from build123d import *

# Parameters (mm, degrees)
F0_W     = 44.8449254036
F0_H     = 34.0256392956
F1_DEPTH = 330
F2_DEPTH = 900
F3_DEPTH = 600
F4_T     = -18
F6_W     = 48.9012300968
F6_H     = 42.5849854946
F7_DEPTH = 330
F8_DEPTH = 700
F9_DEPTH = 600
F10_T    = -18


with BuildPart() as f1:
    # F0 (on Front) → F1 (new body)
    with BuildSketch(Plane.XZ):
        with Locations((22.4224627018, 17.0128196478)):
            Rectangle(F0_W, F0_H)
    extrude(amount=F1_DEPTH)

    # F2 (add): a face of the model
    f2_faces = [f1.faces().sort_by_distance(p)[0] for p in [
        (0, -165, 17.0128196478),
    ]]
    extrude(f2_faces, amount=-F2_DEPTH)

    # F3 (add): a face of the model
    f3_faces = [f1.faces().sort_by_distance(p)[0] for p in [
        (450, -165, 0),
    ]]
    extrude(f3_faces, amount=-F3_DEPTH)

    # F4
    f4_openings = [f1.faces().sort_by_distance(p)[0] for p in [
        (450, -330, 300),
    ]]
    offset(amount=F4_T, openings=f4_openings)


with BuildPart() as f7:
    # F6 (on Front) → F7 (new body)
    with BuildSketch(Plane.XZ):
        with Locations((24.4506150484, 21.2924927473)):
            Rectangle(F6_W, F6_H)
    extrude(amount=F7_DEPTH)

    # F8 (add): a face of the model
    f8_faces = [f7.faces().sort_by_distance(p)[0] for p in [
        (0, -165, 21.2924927473),
    ]]
    extrude(f8_faces, amount=-F8_DEPTH)

    # F9 (add): a face of the model
    f9_faces = [f7.faces().sort_by_distance(p)[0] for p in [
        (350, -165, 0),
    ]]
    extrude(f9_faces, amount=-F9_DEPTH)

    # F10
    f10_openings = [f7.faces().sort_by_distance(p)[0] for p in [
        (350, -330, 300),
    ]]
    offset(amount=F10_T, openings=f10_openings)


solid = f7.part
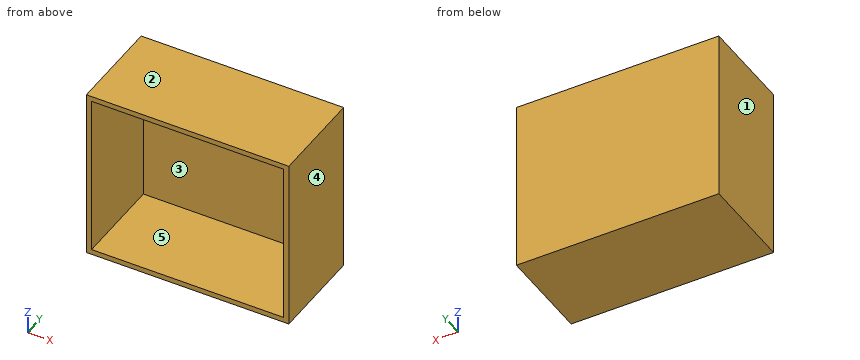
Can you work these out from the model? Positions are in its coordinate system, mm. Face numbers are marked on the shaded views. A direction names the side the tool comes from. Coordinates: 2 decimals unless noted, no trailing zeros. Loops run counter-clockwise (first coordinate to the right, second up) from the corner with the lowest first, then second, coordinate; pieces in that order, holes last. Notation, with made-up numbers: M 84,33.25 L 134,33.25 A30 ccw 134,71.25 Z; hole C 4.25,57 d1. An arc over 180 degrees is marked long. Return JSON: item names as keys, results as strings. Group by question number.
Item 1: Imagine slicing it at A-A (y = -257.5). Please give me the cut outline in (x, z).
Item 2: Thinking about a two-plate mould opening in Z: for the marked faces 1, 2 and 3, which applies, released by +Z, released by -Z, zero draft, split by the parting line, or undercut?
Item 3: Imagine slicing it at B-B (x = 570). Please give me the cut outline in (y, z).
Item 4: If I drill on L1, parallel to X at y = -157, z = 110; L2, parallel to Z at x = 202.5, y = -303.5; L3, parallel to Y at x = 653, z = 478, over which ranges is the centre line in solid material (lowest first)? Write a range as from..to.
Item 5: On a 3-axis mill with a long thin cutter (end or side, diameter ignored), from which of +Z, -Z, +X, -X, +Y, -Y can I reach the whole of each face in a straight line? I mean the marked faces 4 and 5. Say none if no direction works.
Item 6: Imagine slicing it at C-C (z = 411.5). Please give me the cut outline in (x, y).
Verdict:
{
 "1": {"outline": "M 0,0 L 700,0 L 700,600 L 0,600 Z; hole M 18,18 L 682,18 L 682,582 L 18,582 Z"},
 "2": {"face 1": "zero draft", "face 2": "released by +Z", "face 3": "undercut"},
 "3": {"outline": "M -330,0 L 0,0 L 0,600 L -330,600 L -330,582 L -18,582 L -18,18 L -330,18 Z"},
 "4": {"L1": "x = 0..18, 682..700", "L2": "z = 0..18, 582..600", "L3": "y = -18..0"},
 "5": {"face 4": "+Z, -Z, +X, +Y, -Y", "face 5": "-Y"},
 "6": {"outline": "M 0,-330 L 18,-330 L 18,-18 L 682,-18 L 682,-330 L 700,-330 L 700,0 L 0,0 Z"}
}
